from build123d import *

# Parameters (mm, degrees)
SKETCH_1_W             = 94
SKETCH_1_H             = 94
EXTRUDE_1088_DEPTH     = 0.8
FILLET_1_R             = 10
CUT_EXTRUDE_1446_REACH = 68.473
SKETCH_2_R             = 1.6
EXTRUDE_1491_DEPTH     = 3
FILLET_2_R             = 0.5


with BuildPart() as part:
    # 草图1 → Extrude 1088 (new body)
    with BuildSketch(Plane(origin=(0, 0, 0), x_dir=(1, 0, 0), z_dir=(0, 1, 0))):
        Rectangle(SKETCH_1_W, SKETCH_1_H)
    extrude(amount=EXTRUDE_1088_DEPTH)

    # 圆角1
    fillet_1_edges = [part.edges().sort_by_distance(p)[0] for p in [
        (47, 0.4, 47),
        (-47, 0.4, 47),
        (-47, 0.4, -47),
        (47, 0.4, -47),
    ]]
    fillet(fillet_1_edges, radius=FILLET_1_R)

    # 草图2 → Cut-Extrude 1446 (cut, up to next)
    with BuildSketch(Plane(origin=(0, 0.8, 0), x_dir=(1, 0, 0), z_dir=(0, 1, 0)), mode=Mode.PRIVATE) as cut_extrude_1446_sk1:
        with Locations(Location((-39.85, 31.85, 0), (0, 0, 270))):
            Circle(SKETCH_2_R)
    cut_extrude_1446_tool1 = extrude(cut_extrude_1446_sk1.sketch, amount=-CUT_EXTRUDE_1446_REACH, mode=Mode.PRIVATE) & part.part
    # 草图2 → Cut-Extrude 1446 (cut, up to next)
    with BuildSketch(Plane(origin=(0, 0.8, 0), x_dir=(1, 0, 0), z_dir=(0, 1, 0)), mode=Mode.PRIVATE) as cut_extrude_1446_sk2:
        with Locations(Location((39.85, 31.85, 0), (0, 0, 270))):
            Circle(SKETCH_2_R)
    cut_extrude_1446_tool2 = extrude(cut_extrude_1446_sk2.sketch, amount=-CUT_EXTRUDE_1446_REACH, mode=Mode.PRIVATE) & part.part
    # 草图2 → Cut-Extrude 1446 (cut, up to next)
    with BuildSketch(Plane(origin=(0, 0.8, 0), x_dir=(1, 0, 0), z_dir=(0, 1, 0)), mode=Mode.PRIVATE) as cut_extrude_1446_sk3:
        with Locations(Location((39.85, -25, 0), (0, 0, 270))):
            Circle(SKETCH_2_R)
    cut_extrude_1446_tool3 = extrude(cut_extrude_1446_sk3.sketch, amount=-CUT_EXTRUDE_1446_REACH, mode=Mode.PRIVATE) & part.part
    # 草图2 → Cut-Extrude 1446 (cut, up to next)
    with BuildSketch(Plane(origin=(0, 0.8, 0), x_dir=(1, 0, 0), z_dir=(0, 1, 0)), mode=Mode.PRIVATE) as cut_extrude_1446_sk4:
        with Locations(Location((-39.85, -25, 0), (0, 0, 270))):
            Circle(SKETCH_2_R)
    cut_extrude_1446_tool4 = extrude(cut_extrude_1446_sk4.sketch, amount=-CUT_EXTRUDE_1446_REACH, mode=Mode.PRIVATE) & part.part
    add(cut_extrude_1446_tool1.solids().sort_by_distance((-39.85, 0.8, -31.85))[0], mode=Mode.SUBTRACT)
    add(cut_extrude_1446_tool2.solids().sort_by_distance((39.85, 0.8, -31.85))[0], mode=Mode.SUBTRACT)
    add(cut_extrude_1446_tool3.solids().sort_by_distance((39.85, 0.8, 25))[0], mode=Mode.SUBTRACT)
    add(cut_extrude_1446_tool4.solids().sort_by_distance((-39.85, 0.8, 25))[0], mode=Mode.SUBTRACT)

    # 草图4 → Extrude 1491 (add, symmetric)
    with BuildSketch(Plane(origin=(0, 0, 0), x_dir=(0, 0, -1), z_dir=(1, 0, 0))):
        Polygon((-41.145, 0.8), (-30.455, 0.8), (-30.455, 5.98), (-32.8, 2.4), (-38.8, 2.4), (-41.145, 5.98), align=None)
    extrude(amount=EXTRUDE_1491_DEPTH, both=True)

    # 圆角2
    fillet_2_edges = [part.edges().sort_by_distance(p)[0] for p in [
        (0, 5.98, 41.145),
        (0, 5.98, 30.455),
    ]]
    fillet(fillet_2_edges, radius=FILLET_2_R)


solid = part.part
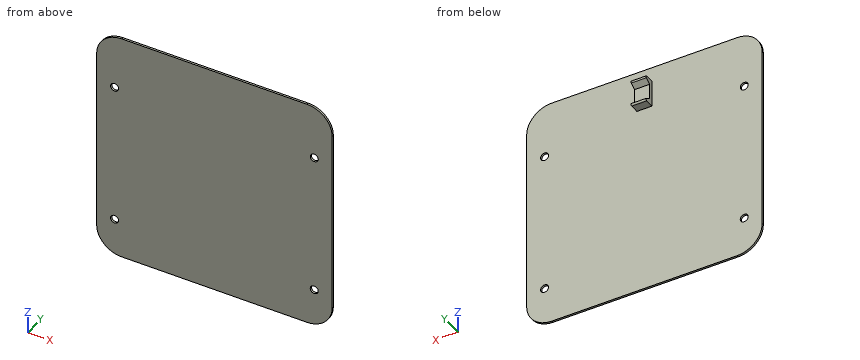
Geometry: final body of the model. Coordinates: model frame, mm. Round coordinates to 2 decimals unless told otherwise and drop trailing zeros. Loops run counter-clockwise (first coordinate to the right, second up) from the corner with the lowest first, then second, coordinate; pieces in that order, holes last. Notation, with made-up numbers: M -22,-34 L -14,-34 A16 ccw -14,-29 Z; hole C -17,84.25 d7. An arc over 180 degrees is marked long. Put each result on its own line as item: value. Start each with the question number.
(1) Material intervals for line 1 along X through (y, z) = (0.65, 25); line 2 along Y through (x, z) = (-40.5, -30); line 3 along X through (y, z) = (0.35, 39.5), sorted ascending. Write a range as [from, to].
(2) Section query A-A (z = -31.85). Return loops of the section in (x, y).
(3) Contact query for flat-ended pins moving along their axis: pin 1 Ø5 at (x, z) = (39.85, -31.85) entering from +Y; pin 2 Ø2 at (y, z) = (2.5, 35.5) entering from -X; pin 3 Ø1.9 at (x, z) = (39.85, 25) entering from -Y; pin 4 Ø1.8 at (x, y) = (1.5, 2) entering from +Z (3 decimals). Output: stop coordinate, or through.
(4) Section query B-B (x = -39.85). Return loops of the section in (y, z).
(5) Section query C-C (x = -17). Return loops of the section in (y, z).
(6) Section query D-D (z = -13). Return loops of the section in (x, y), then the cut area to 3 significant figures.
Findings below:
1. line 1: x = [-47, -41.45], [-38.25, 38.25], [41.45, 47]
1. line 2: y = [0, 0.8]
1. line 3: x = [-46.68, 46.68]
2. outline: M -47,0 L -41.45,0 L -41.45,0.8 L -47,0.8 Z; M -38.25,0 L 38.25,0 L 38.25,0.8 L -38.25,0.8 Z; M 41.45,0 L 47,0 L 47,0.8 L 41.45,0.8 Z
3. pin 1: stops at y = 0.8
3. pin 2: stops at x = -3
3. pin 3: passes through
3. pin 4: stops at z = 41.145
4. outline: M 0,-46.59 L 0.8,-46.59 L 0.8,-33.45 L 0,-33.45 Z; M 0,-30.25 L 0.8,-30.25 L 0.8,23.4 L 0,23.4 Z; M 0,26.6 L 0.8,26.6 L 0.8,46.59 L 0,46.59 Z
5. outline: M 0,-47 L 0.8,-47 L 0.8,47 L 0,47 Z
6. outline: M -47,0 L 47,0 L 47,0.8 L -47,0.8 Z
6. area: 75.2 mm2
